Autodesk Inventor part; units mm, degrees
ref_plane "YZ Plane" through (0, 0, 0) normal (1, 0, 0) x (0, 1, 0)
ref_plane "XZ Plane" through (0, 0, 0) normal (0, 1, 0) x (-1, 0, 0)
ref_plane "XY Plane" through (0, 0, 0) normal (0, 0, 1) x (1, 0, 0)
sketch "Sketch1" plane through (0, 0, 0) normal (0, 0, 1) x (1, 0, 0)
  line L0 (0, 0) -> (5, 0)
  line L1 (5, 0) -> (5, 5)
  line L2 (5, 5) -> (50, 5)
  line L3 (50, 5) -> (50, 0)
  line L4 (50, 0) -> (55, 0)
  line L5 (55, 0) -> (55, 50)
  line L6 (55, 50) -> (0, 50)
  line L7 (0, 50) -> (0, 0)
  dimension "d0" = 50
  dimension "d1" = 5
  dimension "d2" = 5
  dimension "d3" = 5
  dimension "d4" = 45
extrude "Extrusion1" add sketch "Sketch1" along normal blind 55
sketch "Sketch2" plane through (0, 50, 0) normal (0, 1, 0) x (1, 0, 0)
  circle A0 centre (27.5, -27.5) radius 10.5
  line L0 (55, -55) -> (0, -55)
  line L1 (0, 0) -> (0, -55)
  dimension "d7" = 21
  dimension "d8" = 27.5
  dimension "d9" = 27.5
extrude "Extrusion2" add sketch "Sketch2" along normal blind 10
sketch "Sketch3" plane through (55, 0, 0) normal (1, 0, 0) x (0, 0, -1)
  line L0 (0, 50) -> (0, 0)
  line L1 (0, 0) -> (0, 35)
  line L2 (0, 35) -> (-35, 10)
  line L3 (-35, 10) -> (-35, 0)
  line L4 (0, 0) -> (-55, 0)
  line L5 (-35, 0) -> (0, 0)
  line L6 (0, 0) -> (0, 35)
  point P0 (-35, 0)
  dimension "d12" = 35
  dimension "d13" = 0
  dimension "d14" = 10
  dimension "d15" = 35
extrude "Extrusion3" add sketch "Sketch3" along normal blind 40
fillet "Fillet1" radius 5 1 edges at (95, 5, 35)
fillet "Fillet2" radius 5 1 edges at (95, 17.5, 0)
properties part number "khurramf_Graphics2"
CAD build for the part. Positions are in the model's coordinates, mm. A direction names the side the tool comes from. Give positions to 0.01 mm unless a question says otherwise; leave off trailing zeros. Order: outer loops, then holes, each group sorted by start corner. A loop starts at its lowest first (then second) coordinate and runs counter-clockwise, first axis right, second up. Notation, with made-up numbers: (73.5, -3) -> (91.5, -3) arc R18 ccw to (91.5, 7) -> close; hole circle Ø7 at (77, 18). An arc over 180 degrees is marked (long way). Return JSON: item names as keys, results as strings.
Q1. Saw through at D-D (z = 12). Write the cut outline in (x, y).
Working result:
{"outline": "(0, 0) -> (5, 0) -> (5, 5) -> (50, 5) -> (50, 0) -> (95, 0) -> (95, 26.43) -> (55, 26.43) -> (55, 50) -> (0, 50) -> close"}
Q2. Saw through at C-C (x = 27.5). Write the cut outline in (y, z).
Working result:
{"outline": "(5, 0) -> (50, 0) -> (50, 17) -> (60, 17) -> (60, 38) -> (50, 38) -> (50, 55) -> (5, 55) -> close"}
Q3. Drill centre lines: line 1 (Y direction, x = 19, z = 25.5); line 2 (Y direction, x = 48.5, z = 20); line 3 (X direction, y = 39, z = 38.5). Where is each one in solid material? Low to high.
Working result:
{"line 1": "5 to 60", "line 2": "5 to 50", "line 3": "0 to 55"}
Q4. Flat gauge pins, fed straight in: pin 1 (5 mm diameter, centred on y = 51.5, z = 10, fed in from +X); pin 2 (8 mm diameter, centred on x = 79, y = 6.5, fed in from +Z); pin 3 (2 mm diameter, centred on x = 37.5, z = 34, fed in from -Y). Where does each tip first touch, or does it go through?
Working result:
{"pin 1": "x = 55", "pin 2": "z = 35", "pin 3": "y = 5"}
Q5. Mould opens along X. For faces 1 (the face through (94, 5, 33)), 2 (the face through (27, 25, 55)), 3 (the face through (27, 5, 27)), 4 (the face through (5, 2, 27)) say: pulls with the +X half, pulls with the -X half, needs draft (parallel to the pull), parting line crosses it, or undercut.
Working result:
{"face 1": "pulls with the +X half", "face 2": "needs draft", "face 3": "undercut", "face 4": "undercut"}
Q6. Saw through at B-B (y = 15). Write the cut outline in (x, z).
Working result:
{"outline": "(0, 0) -> (90, 0) arc R5 ccw to (95, 5) -> (95, 28) -> (55, 28) -> (55, 55) -> (0, 55) -> close"}
Q7. Which spindle directions (+Z, -Z, +X, -X, +Y, -Y) get a long thin tool onto all of the face, cutting with end or side? Do faces 5 (the face through (74.72, 22.675, 17.255)), 6 (the face through (72, 5, 35)), 7 (the face through (40, 50, 27)). Say none if no direction does.
Working result:
{"face 5": "+Z, +X, +Y", "face 6": "+Z, +X, +Y, -Y", "face 7": "+Y"}
Q8. Saw through at A-A (z = 42.5). Write the cut outline in (x, y), then the cut area to 4 significant figures.
Working result:
{"outline": "(0, 0) -> (5, 0) -> (5, 5) -> (50, 5) -> (50, 0) -> (55, 0) -> (55, 50) -> (0, 50) -> close", "area": "2,525 mm²"}
